```python
from build123d import *

# Parameters (mm, degrees)
SKETCH_1_W             = 41.5
SKETCH_1_H             = 21
EXTRUDE_1_DEPTH        = 4
FILLET_1_R             = 2
FILLET_2_R             = 0.5
SKETCH_2_W             = 28.5
SKETCH_2_H             = 14
EXTRUDE_2_DEPTH        = 3
FILLET_3_R             = 0.5
SKETCH_3_W             = 36
SKETCH_3_H             = 17.5
EXTRUDE_3_DEPTH        = 12
CHAMFER_1_SIZE         = 6
CHAMFER_1_SIZE2        = 2.671372112
CHAMFER_1_PART_2_SIZE  = 6
CHAMFER_1_PART_2_SIZE2 = 2.671372112
SKETCH_4_W             = 1
SKETCH_4_H             = 5
EXTRUDE_4_DEPTH        = 9
FILLET_4_R             = 1
SKETCH_5_R             = 0.75
CUT_EXTRUDE_1_DEPTH    = 21


with BuildPart() as part:
    # Эскиз1 → Бобышка-Вытянуть1 (new body)
    with BuildSketch(Plane(origin=(0, 0, 0), x_dir=(1, 0, 0), z_dir=(0, 1, 0))):
        Rectangle(SKETCH_1_W, SKETCH_1_H)
    extrude(amount=EXTRUDE_1_DEPTH)

    # Скругление1
    fillet_1_edges = [part.edges().sort_by_distance(p)[0] for p in [
        (20.75, 2, 10.5),
        (-20.75, 2, 10.5),
        (-20.75, 2, -10.5),
        (20.75, 2, -10.5),
    ]]
    fillet(fillet_1_edges, radius=FILLET_1_R)

    # Скругление2
    fillet_2_edges = [part.edges().sort_by_distance(p)[0] for p in [
        (-20.75, 4, 0),
        (0, 4, -10.5),
        (20.75, 4, 0),
        (0, 4, 10.5),
        (-20.164213562, 4, 9.914213562),
        (20.164213562, 4, 9.914213562),
        (20.164213562, 4, -9.914213562),
        (-20.164213562, 4, -9.914213562),
    ]]
    fillet(fillet_2_edges, radius=FILLET_2_R)

    # Эскиз2 → Бобышка-Вытянуть2 (add)
    with BuildSketch(Plane(origin=(0, 4, 0), x_dir=(1, 0, 0), z_dir=(0, 1, 0))):
        Rectangle(SKETCH_2_W, SKETCH_2_H)
    extrude(amount=EXTRUDE_2_DEPTH)

    # Скругление3
    fillet_3_edges = [part.edges().sort_by_distance(p)[0] for p in [
        (14.25, 5.5, 7),
        (14.25, 5.5, -7),
        (-14.25, 5.5, -7),
        (-14.25, 5.5, 7),
        (14.25, 7, 0),
        (0, 7, -7),
        (-14.25, 7, 0),
        (0, 7, 7),
    ]]
    fillet(fillet_3_edges, radius=FILLET_3_R)

    # Эскиз3 → Бобышка-Вытянуть3 (add)
    with BuildSketch(Plane.XZ):
        Rectangle(SKETCH_3_W, SKETCH_3_H)
    extrude(amount=EXTRUDE_3_DEPTH)

    # Фаска1
    chamfer_1_edges = [part.edges().sort_by_distance(p)[0] for p in [
        (18, -12, 0),
    ]]
    chamfer_1_side = [part.faces().sort_by_distance(p)[0] for p in [
        (18, -6, 0),
    ]]
    chamfer(chamfer_1_edges, length=CHAMFER_1_SIZE, length2=CHAMFER_1_SIZE2, reference=chamfer_1_side[0])

    # Фаска1 part 2
    chamfer_1_part_2_edges = [part.edges().sort_by_distance(p)[0] for p in [
        (-18, -12, 0),
    ]]
    chamfer_1_part_2_side = [part.faces().sort_by_distance(p)[0] for p in [
        (-18, -6, 0),
    ]]
    chamfer(chamfer_1_part_2_edges, length=CHAMFER_1_PART_2_SIZE, length2=CHAMFER_1_PART_2_SIZE2, reference=chamfer_1_part_2_side[0])

    # Эскиз4 → Бобышка-Вытянуть4 (add)
    with BuildSketch(Plane.XZ.offset(12)):
        Polygon((13.5, 0.75), (15, 0.75), (15, -7.25), (-15, -7.25), (-15, 0.75), (-13.5, 0.75), (-13.5, -5.75), (13.5, -5.75), align=None)
        with Locations((5, 0.75)):
            Rectangle(SKETCH_4_W, SKETCH_4_H)
        with Locations((0, 0.75)):
            Rectangle(SKETCH_4_W, SKETCH_4_H)
        with Locations((10, 0.75)):
            Rectangle(SKETCH_4_W, SKETCH_4_H)
        with Locations((-5, 0.75)):
            Rectangle(SKETCH_4_W, SKETCH_4_H)
        with Locations((-10, 0.75)):
            Rectangle(SKETCH_4_W, SKETCH_4_H)
    extrude(amount=EXTRUDE_4_DEPTH)

    # Скругление4
    fillet_4_edges = [part.edges().sort_by_distance(p)[0] for p in [
        (5, -21, -1.75),
        (5, -21, 3.25),
        (0, -21, 3.25),
        (0, -21, -1.75),
        (10, -21, -1.75),
        (10, -21, 3.25),
        (-5, -21, -1.75),
        (-5, -21, 3.25),
        (-10, -21, -1.75),
        (-10, -21, 3.25),
    ]]
    fillet(fillet_4_edges, radius=FILLET_4_R)

    # Эскиз5 → Вырез-Вытянуть1 (cut)
    with BuildSketch(Plane.ZY.offset(10.5)):
        with Locations((0.75, -18.5)):
            Circle(SKETCH_5_R)
    extrude(amount=-CUT_EXTRUDE_1_DEPTH, mode=Mode.SUBTRACT)


solid = part.part
```
Check sheet for the modelled part. Datum: model origin and axes. Units: mm. A direction names the side the tool comes from. Coordinates: 2 decimals unless noted, no trailing zeros. Order: outer loops, then holes, each group sorted by start corner. A loop starts at its lowest first (then second) coordinate and runs counter-clockwise, first axis right, second up. Notation, with made-up numbers: (-30, 37) -> (-13, 37) arc R25 cw to (-13, 72) -> close; hole circle Ø6 at (88.25, 70.5). An arc over 180 degrees is marked (long way). Write item = value, one per line. Start each with the question number.
1) Material ranges on L1, parallel to Z at x = -5, y = -14.25; L2, parallel to Y at x = -0.05, z = 0.75; L3, parallel to X at y = -18.5, z = -5.25, recorded low to high.
2) Cross-section at D-D (y = -3.75). Enter the section's corners in (x, z), then the cut area to 3 significant figures.
3) Cross-section at A-A (x = 6). Enter the section's corners in (y, z).
4) Mould release check, pull along Z, two halves, no side actions. Record for faces 4 (the flat face through (-4.5, -16, 1)), 5 (the cylindrical face through (-4.993, -20.699, -1.465)), 6 (the cylindrical face through (5.007, -20.699, 2.965)): +Z half, -Z half, draft (parallel to the pull), parting line (faces both ways), or undercut.
5) Access from +Z, -Z, +X, -X, +Y, -Y to the whole of each face (thin tool, end or side, straight path). Record for faces 1 (the flat face through (10.5, -16, 1)), 2 (the flat face through (5, -16, 3.25)), 3 (the flat face through (5, -16, -1.75)).
6) Go/stop test with flat-tipped pins: P1, Ø1, axis at y = -5.5, z = -2, coming from the +X side; P2, Ø1.5, axis at x = 5, y = -15.5, coming from the +Z side; P3, Ø2.5, axis at y = -18.5, z = 0, coming from the +X side. Record where each tip stops, or that it passes through.
7) Cross-section at C-C (y = -18.5). State how many separate pieces and enclosed holes the cut face has, then the cut area to 3 significant figures.
8) Cross-section at B-B (z = -3). Enter the section's corners in (x, y).
Ans:
q1.L1 = -7.25 to -5.75, -1.75 to 3.25
q1.L2 = -21 to -19.25, -17.75 to 7
q1.L3 = -15 to -13.5, 13.5 to 15
q2.outline = (-18, -8.75) -> (18, -8.75) -> (18, 8.75) -> (-18, 8.75) -> close
q2.area = 630 mm²
q3.outline = (-21, -7.25) -> (-12, -7.25) -> (-12, -8.75) -> (0, -8.75) -> (0, -10.5) -> (3.5, -10.5) arc R0.5 ccw to (4, -10) -> (4, -7) -> (6.5, -7) arc R0.5 ccw to (7, -6.5) -> (7, 6.5) arc R0.5 ccw to (6.5, 7) -> (4, 7) -> (4, 10) arc R0.5 ccw to (3.5, 10.5) -> (0, 10.5) -> (0, 8.75) -> (-12, 8.75) -> (-12, -5.75) -> (-21, -5.75) -> close
q4.face_4 = draft
q4.face_5 = undercut
q4.face_6 = +Z half
q5.face_1 = +Z, -Y
q5.face_2 = +Z, +X, -X, -Y
q5.face_3 = -Y
q6.P1 = 18
q6.P2 = 3.25
q6.P3 = 15
q7.separate_pieces = 11
q7.enclosed_holes = 0
q7.area = 82.0 mm²
q8.outline = (-20.75, 0) -> (-18, 0) -> (-18, -6) -> (-15.33, -12) -> (-15, -12) -> (-15, -21) -> (-13.5, -21) -> (-13.5, -12) -> (13.5, -12) -> (13.5, -21) -> (15, -21) -> (15, -12) -> (15.33, -12) -> (18, -6) -> (18, 0) -> (20.75, 0) -> (20.75, 3.5) arc R0.5 ccw to (20.25, 4) -> (14.25, 4) -> (14.25, 6.5) arc R0.5 ccw to (13.75, 7) -> (-13.75, 7) arc R0.5 ccw to (-14.25, 6.5) -> (-14.25, 4) -> (-20.25, 4) arc R0.5 ccw to (-20.75, 3.5) -> close
